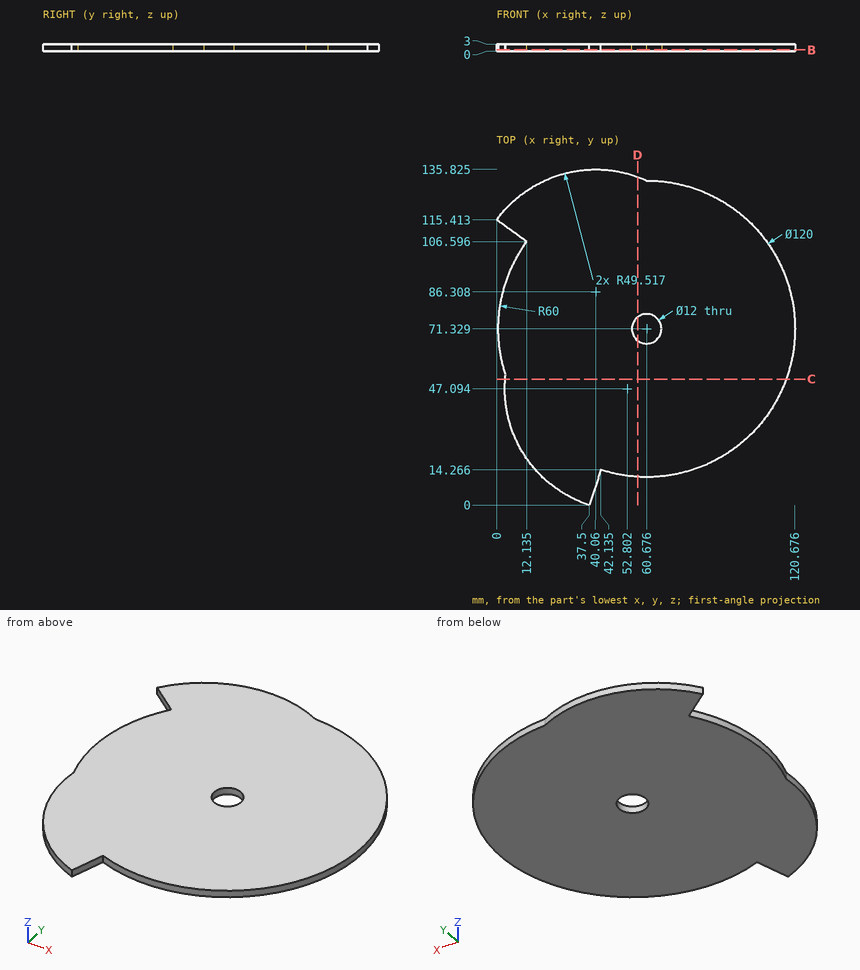
The drawing under review shows one solid part. Ordinate dimensions are in mm from its lowest x, y, z. Give positions to 0.01 mm unless a question says otherwise; leave off trailing zeros. Write each loop counter-clockwise with the first axis right and the second up, starting at its lowest first coordinate (ties: lowest second). Pieces come first, ordered by that corner, then holes.
1. Wall thickness on L1, parallel to Y at x = 65, z = 1.85 (1 decimal); L2, parallel to X at y = 76, z = 2.4 (1 decimal); L3, parallel to X at y = 39, z = 1.9: over which ranges is each line inside the solid? List them lowest first.
2. Add section C-C, the plane y = 51. Write out the cut boundary in (x, z), plus the area to 3 significant figures.
3. For P1, Ø1.5, axis at y = 25.5, z = 0.5, coming from the +X side, flat-tipped, find the tip position at first contact; note if it passes through.
4. Add section B-B, the plane z = 0.65. Write out the cut boundary in (x, y) (1 decimal), plus the area to 3 significant figures.
5. Add section D-D, the plane x = 57. Write out the cut boundary in (y, z).
Worked answers:
1. L1: y = 11.5 to 67.2, 75.5 to 131.2
1. L2: x = 0.9 to 56.9, 64.4 to 120.5
1. L3: x = 3.95 to 111.22
2. outline: (3.44, 0) - (117.13, 0) - (117.13, 3) - (3.44, 3) - close
2. area: 341 mm2
3. P1: stops at x = 100.27
4. outline: (0, 115.4) - (12.1, 106.6) arc R60 ccw to (3.6, 52.8) arc R49.5 ccw to (37.5, 0) - (42.1, 14.3) arc R60 ccw (long way) to (60.7, 131.3) arc R49.5 ccw to start; hole circle Ø12 at (60.7, 71.3)
4. area: 12,400 mm2
5. outline: (11.44, 0) - (66.59, 0) - (66.59, 3) - (11.44, 3) - close; (76.07, 0) - (132.84, 0) - (132.84, 3) - (76.07, 3) - close
